The listing builds one solid part. Answer for the finished solid, in the listing's coordinates (mm). A direction names the side the tool comes from. Round coordinates to 2 decimals unless told otherwise and drop trailing zeros. Write each loop counter-clockwise with the first axis right and the second up, starting at its lowest first coordinate (ties: lowest second). Pieces come first, ordered by that corner, then holes.
(1) A cutting plane is placed at C-C, the plane y = 13.5. Give the vertices of the cut face in (x, z), and give its area (3 significant figures).
(2) Find the intervals of material crossed by probe 1 along Z at (x, y) = (0, 10.5); probe 2 along X at (y, z) = (-7, 635); probe 3 along Z at (x, y) = (22, -35.5), in increasing order.
(3) The mould has two halves that part along Z. Classify faces 5 (the face through (19, -19, 175)), 6 (the face through (20.765, -39.923, 125.7)), 7 (the face through (1, 1, 75)): +Z half, -Z half, draft (parallel to the pull), parting line (faces both ways), or undercut.
(4) A cutting plane is placed at D-D, the plane y = -36. Give the vertices of the cut face in (x, z), and give its area (3 significant figures).
(5) For faces 1 (the face through (9.229, -0.35, 652.743)), 2 (the face through (9, -25, 654)), 3 (the face through (23.846, 7.509, 390.483)), 4 (the face through (9, 25, 654)), determine the directions among +Z, -Z, +X, -X, +Y, -Y from which every point of the face is accessible in a straight line to the end or side of a thin tool.
(6) A cutting plane is placed at A-A, the plane z = 635. Give the vertices of the cut face in (x, y).
(7) A cutting plane is placed at B-B, the plane x = -7.5. Give the vertices of the cut face in (y, z), and give its area (3 significant figures).
(8) Each of these flat-tipped pins is pushed along its axis until it touches: pin 1 Ø5 at (y, z) = (-11, 328) entering from +X; pin 2 Ø5 at (y, z) = (29.5, 135.5) entering from +X; pin 3 Ø24 at (x, z) = (0, 635) entering from -Y; pin 4 Ø5 at (y, z) = (-11.5, 526) entering from +X. Where does it stop, or does it pass through?
from build123d import *

# Parameters (mm, degrees)
SKETCH3_R           = 43
SKETCH3_R_2         = 20
BOSS_EXTRUDE1_DEPTH = 25


with BuildPart() as part:
    # Sketch1 → Revolve1 (revolve)
    with BuildSketch(Plane(origin=(0, 0, 0), x_dir=(1, 0, 0), z_dir=(0, 1, 0))):
        Polygon((0, -75), (45, -75), (45, -175), (25, -175), (25, -600.014288631), (0, -600.014288631), align=None)
    revolve(axis=Axis((0, 0, 75), (0, 0, 1)))

    # Sketch3 → Boss-Extrude1 (add, symmetric)
    with BuildSketch(Plane(origin=(0, 0, 0), x_dir=(1, 0, 0), z_dir=(0, 1, 0))):
        with Locations((0, -635)):
            Circle(SKETCH3_R)
        with Locations((0, -635)):
            Circle(SKETCH3_R_2, mode=Mode.SUBTRACT)
    extrude(amount=BOSS_EXTRUDE1_DEPTH, both=True)


solid = part.part
Solutions:
1. outline: (-42.93, 75) - (42.93, 75) - (42.93, 175) - (21.04, 175) - (21.04, 597.5) arc R43 ccw (long way) to (-21.04, 597.5) - (-21.04, 175) - (-42.93, 175) - close; hole circle Ø40 at (0, 635)
1. area: 30,800 mm2
2. probe 1: z = 75 to 615, 655 to 678
2. probe 2: x = -43 to -20, 20 to 43
2. probe 3: z = 75 to 175
3. face 5: undercut
3. face 6: draft
3. face 7: -Z half
4. outline: (-27, 75) - (27, 75) - (27, 175) - (-27, 175) - close
4. area: 5,400 mm2
5. face 1: +Y, -Y
5. face 2: +Z, +X, -X, -Y
5. face 3: none
5. face 4: +Z, +X, -X, +Y
6. outline: (-43, -25) - (-20, -25) - (-20, 25) - (-43, 25) - close; (20, -25) - (43, -25) - (43, 25) - (20, 25) - close
7. outline: (-44.37, 75) - (44.37, 75) - (44.37, 175) - (23.85, 175) - (23.85, 592.66) - (25, 592.66) - (25, 616.46) - (-25, 616.46) - (-25, 592.66) - (-23.85, 592.66) - (-23.85, 175) - (-44.37, 175) - close; (-25, 653.54) - (25, 653.54) - (25, 677.34) - (-25, 677.34) - close
7. area: 31,200 mm2
8. pin 1: stops at x = 23.51
8. pin 2: stops at x = 36
8. pin 3: passes through
8. pin 4: stops at x = 23.32
